Could you check a few things on this model? Use its own coordinates, in mm. A direction names the side the tool comes from. Coordinates: 2 decimals unless noted, no trailing zeros. Loops run counter-clockwise (first coordinate to the right, second up) from the corner with the lowest first, then second, coordinate; pieces in that order, holes last. Notation, with made-up numbers: (42, -39) -> (70, -39) arc R23 cw to (70, 0) -> close; hole circle Ø8 at (-30, -13). An arc over 180 degrees is marked (long way). One line per question, with ' | ' between items.
```python
from build123d import *

# Parameters (mm, degrees)
F0_W     = 38.1
F0_H     = 44.45
F1_DEPTH = 25.4
F2_R     = 19.04999
F3_R     = 12.7
F4_DEPTH = 25.401
F5_R     = 3.175
F6_DEPTH = 12.7


# Not quite as in the source:
# - a fillet or chamfer is up to 0.001 mm smaller than in the source, because OpenCascade refuses the exact size


with BuildPart() as f1:
    # F0 (on Front) → F1 (new body)
    with BuildSketch(Plane.XZ):
        with Locations((19.05, 22.225)):
            Rectangle(F0_W, F0_H)
    extrude(amount=F1_DEPTH)

    # F2 (radius 19.05 in the source; OpenCascade refuses exactly that, so slightly less here)
    f2_edges = [f1.edges().sort_by_distance(p)[0] for p in [
        (0, -12.7, 44.45),
        (38.1, -12.7, 44.45),
    ]]
    fillet(f2_edges, radius=F2_R)

    # F3 (on face) → F4 (cut, through all)
    with BuildSketch(Plane.XZ.offset(25.4)):
        with Locations((19.05, 25.4)):
            Circle(F3_R)
    extrude(amount=-F4_DEPTH, mode=Mode.SUBTRACT)

    # F5 (on face) → F6 (cut)
    with BuildSketch(Plane(origin=(0, 0, 0), x_dir=(1, 0, 0), z_dir=(0, 0, -1))):
        with Locations((6.35, 12.7)):
            Circle(F5_R)
        with Locations((31.75, 12.7)):
            Circle(F5_R)
    extrude(amount=-F6_DEPTH, mode=Mode.SUBTRACT)


solid = f1.part
```
Q1. Imagine slicing it at B-B on z = 15.5. Write out the boundary of the cut face in (x, y), plus the area to 3 significant figures.
Values follow:
outline: (0, -25.4) -> (11.1, -25.4) -> (11.1, 0) -> (0, 0) -> close; (27, -25.4) -> (38.1, -25.4) -> (38.1, 0) -> (27, 0) -> close | area: 564 mm2
Q2. Imagine slicing it at C-C on x = 26. Write out the boundary of the cut face in (y, z), plus the area to 3 significant figures.
Values follow:
outline: (-25.4, 0) -> (0, 0) -> (0, 14.77) -> (-25.4, 14.77) -> close; (-25.4, 36.03) -> (0, 36.03) -> (0, 43.14) -> (-25.4, 43.14) -> close | area: 556 mm2
Q3. For pin 1 (1.9 mm diameter, centred on x = 33, y = -12.5, fed in from -Z); pin 2 (5 mm diameter, centred on y = -18.5, z = 33.5, fed in from +X); pin 3 (4 mm diameter, centred on x = 31.75, y = -12.7, fed in from +Z), each with a flat end and sliding along its axis, tell me the tip position at first contact or that it passes through.
Values follow:
pin 1: stops at z = 12.7 | pin 2: stops at x = 37.26 | pin 3: stops at z = 41.16
Q4. We'd pull the mould along Y, two halves only. Please class faces 1 (the face through (15, -25.4, 13)), 2 (the face through (6, -13, 12.7)), 3 (the face through (0, -13, 13)), 4 (the face through (31.06, -9.6, 6.26)): released by +Y, released by -Y, zero draft, split by the parting line, or undercut.
Values follow:
face 1: released by -Y | face 2: undercut | face 3: zero draft | face 4: undercut
Q5. Please list where these lines run through material, in increasing order: L1, parallel to X at y = -12.7, z = 9.5 (3 decimals); L2, parallel to Y at x = 31.75, z = 5.25 (3 decimals); L3, parallel to Z at x = 19.05, y = -8.25. Write a range as [from, to].
Values follow:
L1: x = [0, 3.175], [9.525, 28.575], [34.925, 38.1] | L2: y = [-25.4, -15.875], [-9.525, 0] | L3: z = [0, 12.7], [38.1, 44.45]
Q6. For faces 5 (the face through (32, -13, 12.7)), 6 (the face through (5.43, -12.88, 38.72)), which set-ups out of +Z, -Z, +X, -X, +Y, -Y let a thin tool reach every point of the face, with its end or its side?
Values follow:
face 5: -Z | face 6: +Z, -X, +Y, -Y
Q7. Imagine slicing it at D-D on x = 4. Write out the boundary of the cut face in (y, z), plus the area to 3 significant figures.
Values follow:
outline: (-25.4, 0) -> (-14.83, 0) -> (-14.83, 12.7) -> (-10.57, 12.7) -> (-10.57, 0) -> (0, 0) -> (0, 37.08) -> (-25.4, 37.08) -> close | area: 888 mm2
